The listing builds one solid part. Answer for the finished solid, in the listing's coordinates (mm). A direction names the side the tool comes from. Coordinates: 2 decimals unless noted, no trailing zeros. Loops run counter-clockwise (first coordinate to the right, second up) from the corner with the lowest first, then second, coordinate; pieces in that order, holes last. Notation, with made-up numbers: (64.5, 45.25) -> (101.5, 45.25) arc R23 ccw to (101.5, 60.25) -> close; hole circle Ø6 at (-31, 73). An arc over 180 degrees is marked (long way). Answer in a Markdown table with one row per item.
Autodesk Inventor part; units mm, degrees
ref_plane "YZ Plane" through (0, 0, 0) normal (1, 0, 0) x (0, 1, 0)
ref_plane "XZ Plane" through (0, 0, 0) normal (0, 1, 0) x (-1, 0, 0)
ref_plane "XY Plane" through (0, 0, 0) normal (0, 0, 1) x (1, 0, 0)
sketch "Sketch1" plane through (0, 0, 0) normal (0, 0, 1) x (1, 0, 0)
  circle A0 centre (0.25, 36.05) radius 28
  line L0 (-21, -56.05) -> (-21, -1.05)
  line L1 (-21, -1.05) -> (21.5, -1.05)
  line L2 (21.5, -1.05) -> (21.5, -56.05)
  line L3 (21.5, -56.05) -> (-21, -56.05)
  arc A1 (-41, -66.05) -> (-36, -71.05) centre (-36, -66.05) ccw
  line L4 (-36, -71.05) -> (36, -71.05)
  arc A2 (36, -71.05) -> (41, -66.05) centre (36, -66.05) ccw
  line L5 (41, -66.05) -> (41, 71.05)
  line L6 (41, 71.05) -> (-41, 71.05)
  line L7 (-41, 71.05) -> (-41, -66.05)
  line L8 (20, 69.05) -> (20, 73.05)
  line L9 (20, 69.05) -> (33.3542, 69.05)
  arc A3 (33.3542, 69.05) -> (39, 63.4042) centre (36, 66.05) ccw
  line L10 (39, 63.4042) -> (39, -63.4042)
  arc A4 (39, -63.4042) -> (33.3542, -69.05) centre (36, -66.05) ccw
  line L11 (33.3542, -69.05) -> (-33.3542, -69.05)
  arc A5 (-33.3542, -69.05) -> (-39, -63.4042) centre (-36, -66.05) ccw
  line L12 (-39, -63.4042) -> (-39, 63.4042)
  arc A6 (-39, 63.4042) -> (-33.3542, 69.05) centre (-36, 66.05) ccw
  line L13 (-33.3542, 69.05) -> (-20, 69.05)
  line L14 (-20, 69.05) -> (-20, 73.05)
  line L15 (-39, 73.05) -> (-20, 73.05)
  line L16 (-39, 79.0505) -> (-39, 73.05)
  arc A7 (-34, 89.95) -> (-39, 84.95) centre (-34, 84.95) ccw
  line L17 (34, 89.95) -> (-34, 89.95)
  arc A8 (39, 84.95) -> (34, 89.95) centre (34, 84.95) ccw
  line L18 (39, 73.05) -> (39, 79.0505)
  line L19 (20, 73.05) -> (39, 73.05)
  line L20 (41, -66.05) -> (41, 86.95)
  arc A9 (41, 86.95) -> (36, 91.95) centre (36, 86.95) ccw
  line L21 (-36, 91.95) -> (36, 91.95)
  arc A10 (-36, 91.95) -> (-41, 86.95) centre (-36, 86.95) ccw
  line L22 (-41, -66.05) -> (-41, 86.95)
  arc A11 (-41, -66.05) -> (-36, -71.05) centre (-36, -66.05) ccw
  line L23 (-36, -71.05) -> (36, -71.05)
  arc A12 (36, -71.05) -> (41, -66.05) centre (36, -66.05) ccw
  circle A13 centre (-36, -66.05) radius 2.1
  line L24 (38.6458, 69.05) -> (39, 69.05)
  line L25 (39, 69.05) -> (39, 68.6958)
  arc A14 (39, 68.6958) -> (38.6458, 69.05) centre (36, 66.05) ccw
  circle A15 centre (36, 66.05) radius 2.1
  line L26 (39, -68.6958) -> (39, -69.05)
  line L27 (39, -69.05) -> (38.6458, -69.05)
  arc A16 (38.6458, -69.05) -> (39, -68.6958) centre (36, -66.05) ccw
  circle A17 centre (36, -66.05) radius 2.1
  arc A18 (-39, -68.6958) -> (-38.6458, -69.05) centre (-36, -66.05) ccw
  line L28 (-38.6458, -69.05) -> (-39, -69.05)
  line L29 (-39, -69.05) -> (-39, -68.6958)
  circle A19 centre (-36, 66.05) radius 2.1
  arc A20 (-38.6458, 69.05) -> (-39, 68.6958) centre (-36, 66.05) ccw
  line L30 (-39, 68.6958) -> (-39, 69.05)
  line L31 (-39, 69.05) -> (-38.6458, 69.05)
  line L32 (41, 71.25) -> (-41, 71.25)
  circle A21 centre (-36.5, 81.5) radius 2.1
  circle A22 centre (36.5, 81.5) radius 2.1
  arc A23 (-39, 79.0505) -> (-39, 83.9495) centre (-36.5, 81.5) ccw
  line L33 (-39, 84.95) -> (-39, 83.9495)
  line L34 (39, 83.9495) -> (39, 84.95)
  arc A24 (39, 83.9495) -> (39, 79.0505) centre (36.5, 81.5) ccw
  point P0 (0, 0)
  dimension "d0" = 0.2
extrude "Extrusion1" add sketch "Sketch1" along normal blind 2 contours L22 A10 L21 A9 L20 L32 L8 L19 L18 A24 L34 A8 L17 A7 L33 A23 L16 L15 L14 | L14 L15 L16 A23 L33 A7 L17 A8 L34 A24 L18 L19 L8 L32 | A21 | A22
sketch "Sketch2" plane through (0, 0, 0) normal (0, 0, -1) x (-1, 0, 0)
  arc A0 (-34, 89.95) -> (-39, 79.0505) centre (-34, 84.95) ccw
  line L0 (-34, 89.95) -> (34, 89.95)
  arc A1 (39, 79.0505) -> (34, 89.95) centre (34, 84.95) ccw
  line L1 (39, 79.0505) -> (39, 73.05)
  line L2 (-39, 73.05) -> (-39, 79.0505)
  line L3 (38.9, 73.05) -> (38.9, 84.95)
  arc A2 (38.9, 84.95) -> (34, 89.85) centre (34, 84.95) ccw
  line L4 (34, 89.85) -> (-34, 89.85)
  arc A3 (-34, 89.85) -> (-38.9, 84.95) centre (-34, 84.95) ccw
  line L5 (-38.9, 84.95) -> (-38.9, 73.05)
  line L6 (-37.9, 73.05) -> (-37.9, 84.95)
  arc A4 (-34, 88.85) -> (-37.9, 84.95) centre (-34, 84.95) ccw
  line L7 (-34, 88.85) -> (34, 88.85)
  arc A5 (37.9, 84.95) -> (34, 88.85) centre (34, 84.95) ccw
  line L8 (37.9, 84.95) -> (37.9, 73.05)
  line L9 (-38.9, 73.05) -> (-37.9, 73.05)
  line L10 (37.9, 73.05) -> (38.9, 73.05)
  line L11 (41, 71.25) -> (-41, 71.25)
  arc A6 (-34, 89.95) -> (-39, 84.95) centre (-34, 84.95) ccw
  line L12 (-34, 89.95) -> (34, 89.95)
  circle A7 centre (-36.5, 81.5) radius 2.1
  arc A8 (-39, 79.0505) -> (-39, 83.9495) centre (-36.5, 81.5) ccw
  circle A9 centre (36.5, 81.5) radius 2.1
  arc A10 (39, 83.9495) -> (39, 79.0505) centre (36.5, 81.5) ccw
  arc A11 (-36, 91.95) -> (-41, 86.95) centre (-36, 86.95) ccw
  line L13 (-41, 71.25) -> (-41, 86.95)
  line L14 (-34, 88.85) -> (-34, 89.95)
  line L15 (-38.9, 77.05) -> (38.9, 77.05)
  line L16 (34, 89.95) -> (34, 88.85)
  point P0 (0, 0)
  point P1 (-38.4, 73.05)
  point P2 (38.4, 73.05)
  point P3 (-37.9, 83.0652)
  point P4 (-38.3525, 82.4891)
  point P5 (-37.9, 81.8211)
  point P6 (38.3525, 82.4891)
  point P7 (37.9, 83.0652)
  point P8 (37.9, 81.8211)
  point P9 (-37.9, 77.05)
  point P10 (37.9, 77.05)
  point P11 (34, 89.85)
  dimension "d3" = 0.1
  dimension "d4" = 1
  dimension "d5" = 16.8
  dimension "d6" = 16.8
  dimension "d15" = 2.1
  dimension "d16" = 4
extrude "Extrusion2" add sketch "Sketch2" along normal blind 3 contours L4 L16 L7 L14 | L3 L10 L8 L15 | L15 L6 L9 L5
sketch "Sketch3" plane through (0, 0, 2) normal (0, 0, 1) x (1, 0, 0)
  circle A0 centre (36.5, 81.5) radius 2.1
  circle A1 centre (-36.5, 81.5) radius 2.1
  point P0 (0, 0)
extrude "Extrusion3" cut sketch "Sketch3" against normal blind 3
sketch "Sketch4" plane through (0, 0, 2) normal (0, 0, 1) x (1, 0, 0)
  circle A0 centre (36.5, 81.5) radius 2.1
  circle A1 centre (36.5, 81.5) radius 2.75
  circle A2 centre (-36.5, 81.5) radius 2.1
  circle A3 centre (-36.5, 81.5) radius 2.75
  point P0 (0, 0)
  point P1 (-37.9, 79.9348)
  point P2 (-37.9, 83.0652)
  dimension "d11" = 5.5
  dimension "d12" = 5.5
extrude "Extrusion4" cut sketch "Sketch4" against normal blind 1 contours A0 | A1 | A2 | A3
properties part number "colortop"
Item 1: A cutting plane is placed at C-C, the plane x = 4. Determine the outline of the cut face in (y, z), plus the area to 3 significant figures.
Findings below:
| item | result |
|---|---|
| outline | (71.25, 0) -> (88.85, 0) -> (88.85, -3) -> (89.85, -3) -> (89.85, 0) -> (91.95, 0) -> (91.95, 2) -> (71.25, 2) -> close |
| area | 44.4 mm2 |
Item 2: A tool of negligible diameter and unlimited length cuts with its end or side. For faces 5 (the face through (0, 88.85, -1)), 6 (the face through (0, 89.85, -1)), 7 (the face through (-38.9, 75, -1)), 8 (the face through (-37.9, 75, -1)), 9 (the face through (-39.247, 81.621, 1.507)), from which of +Z, -Z, +X, -X, +Y, -Y can it reach the whole face along a straight path? Write none if from no direction.
Findings below:
| item | result |
|---|---|
| face 5 | -Z, +X, -X, -Y |
| face 6 | -Z, +X, -X, +Y |
| face 7 | -Z, -X, +Y, -Y |
| face 8 | -Z, +Y, -Y |
| face 9 | +Z |
Item 3: Find the intervals of material crossed by probe 1 along X at (y, z) = (73.25, -0.2); probe 2 along Y at (x, z) = (-36.5, 0.6); probe 3 along Y at (x, z) = (-36.5, 1.35), in increasing order.
Findings below:
| item | result |
|---|---|
| probe 1 | x = -38.9 to -37.9, 37.9 to 38.9 |
| probe 2 | y = 71.25 to 79.4, 83.6 to 91.92 |
| probe 3 | y = 71.25 to 78.75, 84.25 to 91.92 |
Item 4: Flat-ended cylindrical pins translate along their axes: pin 1 Ø5 at (x, y) = (36.5, 81.5) entering from +Z; pin 2 Ø1.5 at (x, z) = (6.5, -1) entering from +Y; pin 3 Ø2 at (x, y) = (21, 75.5) entering from -Z. Find the tip coordinate at first contact, or state that the pin passes through.
Findings below:
| item | result |
|---|---|
| pin 1 | stops at z = 1 |
| pin 2 | stops at y = 89.85 |
| pin 3 | stops at z = 0 |
Item 5: Determine the mould class of faces 1 (the face through (1, 71.25, 1)), 2 (the face through (37.9, 75, -1)), 3 (the face through (-37, 79, 1)), 4 (the face through (33.753, 81.621, 1.507)) for opening direction Y: +Y half, -Y half, draft (parallel to the pull), parting line (faces both ways), or undercut.
Findings below:
| item | result |
|---|---|
| face 1 | -Y half |
| face 2 | draft |
| face 3 | undercut |
| face 4 | undercut |
Item 6: A cutting plane is placed at D-D, the plane y = 75.75. Determine the outline of the cut face in (x, z), plus the area to 3 significant figures.
Findings below:
| item | result |
|---|---|
| outline | (-41, 0) -> (-38.9, 0) -> (-38.9, -3) -> (-37.9, -3) -> (-37.9, 0) -> (37.9, 0) -> (37.9, -3) -> (38.9, -3) -> (38.9, 0) -> (41, 0) -> (41, 2) -> (-41, 2) -> close |
| area | 170 mm2 |
Item 7: A cutting plane is placed at A-A, the plane y = 81.5. Determine the outline of the cut face in (x, z), plus the area to 3 significant figures.
Findings below:
| item | result |
|---|---|
| outline | (-41, 0) -> (-38.6, 0) -> (-38.6, 1) -> (-39.25, 1) -> (-39.25, 2) -> (-41, 2) -> close; (-34.4, 0) -> (34.4, 0) -> (34.4, 1) -> (33.75, 1) -> (33.75, 2) -> (-33.75, 2) -> (-33.75, 1) -> (-34.4, 1) -> close; (38.6, 0) -> (41, 0) -> (41, 2) -> (39.25, 2) -> (39.25, 1) -> (38.6, 1) -> close |
| area | 145 mm2 |
Item 8: A cutting plane is placed at B-B, the plane z = -1.55. Determine the outline of the cut face in (x, y), plus the area to 3 significant figures.
Findings below:
| item | result |
|---|---|
| outline | (-38.9, 73.05) -> (-37.9, 73.05) -> (-37.9, 77.05) -> (-38.9, 77.05) -> close; (-34, 88.85) -> (34, 88.85) -> (34, 89.85) -> (-34, 89.85) -> close; (37.9, 73.05) -> (38.9, 73.05) -> (38.9, 77.05) -> (37.9, 77.05) -> close |
| area | 76.0 mm2 |
